For this review, use the dimensioned drawing (mm, ordinates from the lowest corner) and the shaded views. Give positions to 0.01 mm unless a question says otherwise; leave off trailing zeros. Order: outer loops, then holes, each group sorted by start corner. A loop starts at its lowest first (then second) coordinate and runs counter-clockwise, first axis right, second up.
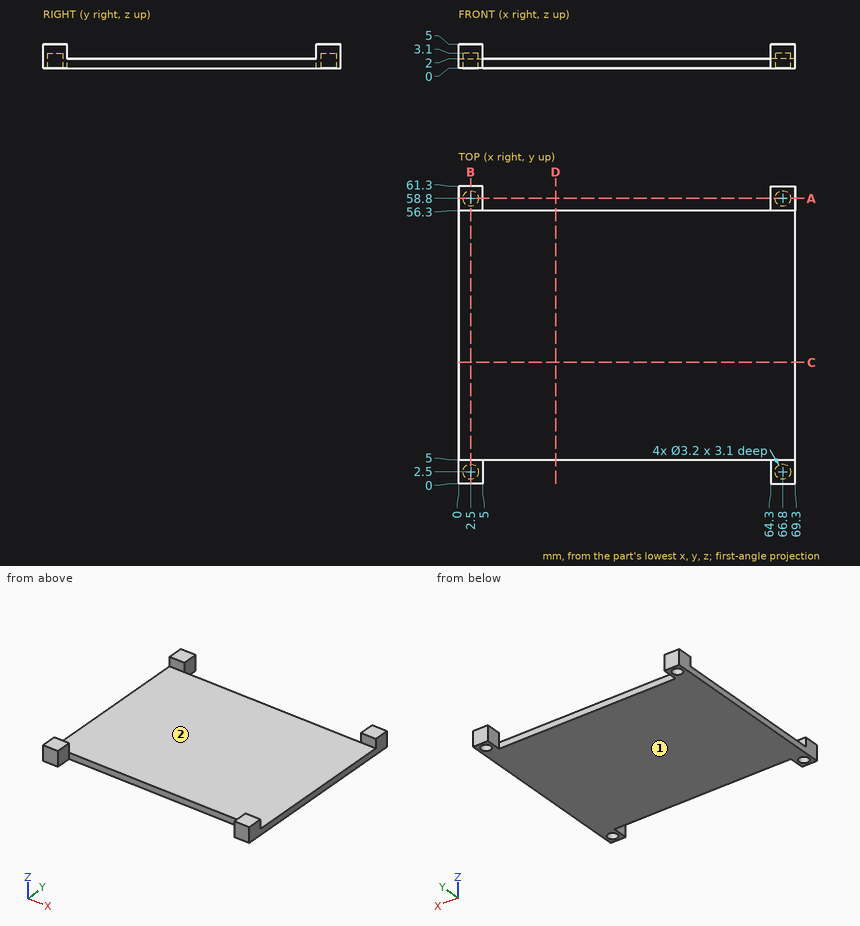
1. Take a section at D-D (x = 20). State the section outline as (y, z) points.
Recorded:
outline: (5, 0) - (56.3, 0) - (56.3, 2) - (5, 2) - close
2. Take a section at A-A (y = 58.8). State the section outline as (x, z) points, then the cut area to 3 significant figures.
Recorded:
outline: (0, 0) - (0.9, 0) - (0.9, 3.1) - (4.1, 3.1) - (4.1, 0) - (5, 0) - (5, 5) - (0, 5) - close; (64.3, 0) - (65.2, 0) - (65.2, 3.1) - (68.4, 3.1) - (68.4, 0) - (69.3, 0) - (69.3, 5) - (64.3, 5) - close
area: 30.2 mm2
3. Take a section at B-B (x = 2.5). State the section outline as (y, z) points.
Recorded:
outline: (0, 0) - (0.9, 0) - (0.9, 3.1) - (4.1, 3.1) - (4.1, 0) - (57.2, 0) - (57.2, 3.1) - (60.4, 3.1) - (60.4, 0) - (61.3, 0) - (61.3, 5) - (56.3, 5) - (56.3, 2) - (5, 2) - (5, 5) - (0, 5) - close
4. Draft analysis for pull direction Y (two halves, no side actions). For the marked faces 1 and 2, state which applies: pulls with the +Y half, pulls with the -Y half, needs draft (parallel to the pull), parting line crosses it, or undercut.
Recorded:
face 1: needs draft
face 2: undercut
5. For line 1 along X through (y, z) = (2.5, 1.55); line 2 along Y through (x, z) = (2.5, 2.35); line 3 along Y through (x, z) = (2.5, 1.8), list the stretches that pass through material, from the lowest coordinate up.
Recorded:
line 1: x = 0 to 0.9, 4.1 to 5, 64.3 to 65.2, 68.4 to 69.3
line 2: y = 0 to 0.9, 4.1 to 5, 56.3 to 57.2, 60.4 to 61.3
line 3: y = 0 to 0.9, 4.1 to 57.2, 60.4 to 61.3
6. Take a section at C-C (y = 25). State the section outline as (x, z) points, then the cut area to 3 significant figures.
Recorded:
outline: (0, 0) - (69.3, 0) - (69.3, 2) - (0, 2) - close
area: 139 mm2
7. For pin 1 (12 mm diameter, centred on x = 18, y = 20.5, fed in from -Z); pin 2 (8 mm diameter, centred on x = 39, y = 22, fed in from +Z); pin 3 (1.6 mm diameter, centred on x = 67, y = 59.5, fed in from -Z); pin 4 (1 mm diameter, centred on x = 27.5, z = 1, fed in from +Y), all flat-tipped, find the tip position at first contact; note any pin that passes through.
Recorded:
pin 1: stops at z = 0
pin 2: stops at z = 2
pin 3: stops at z = 3.1
pin 4: stops at y = 56.3
